Verification items for the finished model (mm, model axes). A direction names the side the tool comes from. Give positions to 0.01 mm unless a question says otherwise; leave off trailing zeros. Loops run counter-clockwise (first coordinate to the right, second up) from the corner with the lowest first, then second, coordinate; pieces in that order, holes last. Notation, with made-up numbers: M 77.5,9.5 L 134.5,9.5 A23 ccw 134.5,41.5 Z; hole C 75,21.5 d7. An arc over 180 degrees is marked long. Answer in a Markdown table with one row per item.
```python
from build123d import *

# Parameters (mm, degrees)
F0_R      = 4
F1_DEPTH  = 10
F3_DEPTH  = 7
F4_R      = 1.8
F9_DEPTH  = 25
F11_DEPTH = 40


with BuildPart() as f1:
    # F0 (on Front) → F1 (new body, symmetric)
    with BuildSketch(Plane.XZ):
        Polygon((0, -20), (0, -25), (100, -25), (100, -9), (38, -9), (38, -20), (30, -20), align=None)
        with BuildLine():
            Line((0, -15), (0, -20))
            Line((0, -20), (30, -20))
            Line((30, -20), (30, -15))
            ThreePointArc((30, -15), (15, 0), (0, -15))
        make_face()
        with Locations((15, -9)):
            Circle(F0_R, mode=Mode.SUBTRACT)
    extrude(amount=F1_DEPTH, both=True)

    # F2 (on Front) → F3 (cut, symmetric)
    with BuildSketch(Plane.XZ):
        with BuildLine():
            Line((30, -20), (30, -15))
            ThreePointArc((30, -15), (15, 0), (0, -15))
            Line((0, -15), (0, -20))
            Line((0, -20), (30, -20))
        make_face()
    extrude(amount=F3_DEPTH, both=True, mode=Mode.SUBTRACT)

    # F4
    f4_edges = [f1.edges().sort_by_distance(p)[0] for p in [
        (15, 7, -20),
        (15, -7, -20),
        (30, -8.5, -20),
        (30, 8.5, -20),
        (38, 0, -9),
    ]]
    fillet(f4_edges, radius=F4_R)

    # F8 (on face) → F9 (cut, symmetric)
    with BuildSketch(Plane(origin=(53.9389180046, 33.7047767362, 0), x_dir=(-0.5299192642, 0.8480480962, 0), z_dir=(0.8480480962, 0.5299192642, 0))):
        Polygon((-38.0182327263, -9), (-43.0182327263, -9), (-43.0182327263, -14), align=None)
    extrude(amount=F9_DEPTH, both=True, mode=Mode.SUBTRACT)

    # F10 (on offset) → F11 (cut, symmetric)
    with BuildSketch(Plane.YZ.offset(75)):
        Polygon((0.5, -9), (0, -9), (-0.5, -9), (-0.5, -19), (0.5, -19), align=None)
    extrude(amount=F11_DEPTH, both=True, mode=Mode.SUBTRACT)


solid = f1.part
```
Item 1: Scan lines: L1, parallel to Y at x = 6, z = -7.5; L2, parallel to Z at x = 15, y = 8.1; L3, parallel to Z at x = 49, y = -7. Record each from-to range of solid material in increasing order. Write a range as [from, to].
Reported:
| item | result |
|---|---|
| L1 | y = [-10, -7], [7, 10] |
| L2 | z = [-25, -13], [-5, 0] |
| L3 | z = [-25, -9] |
Item 2: Sectioned sample at C-C (x = 92.5). Record the cut outline in (y, z).
Reported:
| item | result |
|---|---|
| outline | M -10,-25 L 10,-25 L 10,-11.52 L 7.07,-14 L 7.07,-9 L 0.5,-9 L 0.5,-19 L -0.5,-19 L -0.5,-9 L -10,-9 Z |
Item 3: Tool access check on faces 1 (the flat face through (38, -2, -15)), 2 (the flat face through (85.035, 5.317, -11.535)), 3 (the flat face through (69, -0.5, -14)), 4 (the flat face through (52, -5, -9)). Record the directions out of +Z, -Z, +X, -X, +Y, -Y that give a thin tool (end or side, any length) a straight path to the whole face; none if there is none.
Reported:
| item | result |
|---|---|
| face 1 | +Z, +Y, -Y |
| face 2 | +Z |
| face 3 | +Z, +X, -X |
| face 4 | +Z, +X, +Y, -Y |
Item 4: Go/stop test with flat-tipped pins: pin 1 (0.8 mm diameter, centred on x = 80, y = 0, fed in from +Z); pin 2 (6.5 mm diameter, centred on x = 15, z = -9, fed in from -Y); pin 3 (4 mm diameter, centred on x = 70, y = 7.5, fed in from +Z); pin 4 (10 mm diameter, centred on x = 28, y = -4.5, fed in from +Z). Record where each tip stops, or that it passes through.
Reported:
| item | result |
|---|---|
| pin 1 | stops at z = -19 |
| pin 2 | passes through |
| pin 3 | stops at z = -9 |
| pin 4 | stops at z = -2.76 |
Item 5: Sectioned sample at A-A (x = 15). Record the cut outline in (y, z), and give its area (3 significant figures).
Reported:
| item | result |
|---|---|
| outline | M -10,-25 L 10,-25 L 10,-13 L 7,-13 L 7,-18.2 A1.8 cw 5.2,-20 L -5.2,-20 A1.8 cw -7,-18.2 L -7,-13 L -10,-13 Z; M -10,-5 L -7,-5 L -7,0 L -10,0 Z; M 7,-5 L 10,-5 L 10,0 L 7,0 Z |
| area | 173 mm^2 |
Item 6: Release check for a two-part mould opening along X. For faces 5 (the flat face through (49, 0, -25)), 6 (the flat face through (100, -2, -17)), 7 (the cylindrical face through (38.541, 5.184, -9.513)) record: released by +X, released by -X, zero draft, split by the parting line, or undercut.
Reported:
| item | result |
|---|---|
| face 5 | zero draft |
| face 6 | released by +X |
| face 7 | undercut |
Item 7: Sectioned sample at B-B (x = 77.5). Record the cut outline in (y, z).
Reported:
| item | result |
|---|---|
| outline | M -10,-25 L 10,-25 L 10,-9 L 3.6,-9 L 0.5,-11.63 L 0.5,-19 L -0.5,-19 L -0.5,-12.47 L -2.3,-14 L -2.3,-9 L -10,-9 Z |
